```python
from build123d import *

# Parameters (mm, degrees)
SKETCH1_W                = 114.3
SKETCH1_H                = 101.6
BOSS_EXTRUDE1_DEPTH      = 3.175
F_5_16_CLEARANCE_HOLE2_D = 8.4328


with BuildPart() as part:
    # Sketch1 → Boss-Extrude1 (new body)
    with BuildSketch(Plane(origin=(0, 0, 0), x_dir=(1, 0, 0), z_dir=(0, 1, 0))):
        Rectangle(SKETCH1_W, SKETCH1_H)
    extrude(amount=BOSS_EXTRUDE1_DEPTH)

    # 5/16 Clearance Hole2 (through all)
    with Locations(Plane(origin=(0, 3.175, 0), x_dir=(1, 0, 0), z_dir=(0, 1, 0))):
        with Locations((-38.1, 31.75), (-38.1, 0), (-38.1, -34.925)):
            f_5_16_clearance_hole2 = Hole(F_5_16_CLEARANCE_HOLE2_D / 2)

    # Mirror2: 5/16 Clearance Hole2 across plane
    add(f_5_16_clearance_hole2.mirror(Plane(origin=(0, 0, 0), x_dir=(0, 0, 1), z_dir=(1, 0, 0))), mode=Mode.SUBTRACT)


solid = part.part
```
Build history of the part. All positions in model axes, mm. Round coordinates to 2 decimals unless told otherwise and drop trailing zeros. Order: outer loops, then holes, each group sorted by start corner. A loop starts at its lowest first (then second) coordinate and runs counter-clockwise, first axis right, second up. Notation, with made-up numbers: (-35, -26.75) -> (-13, -26.75) arc R19 ccw to (-13, -8.75) -> close; hole circle Ø3 at (53.25, 86.5). An arc over 180 degrees is marked (long way). Answer in a Markdown table with one row per item.
1) Wall check: L1, parallel to Z at x = -38.1, y = 2.1; L2, parallel to X at y = 2.1, z = -28.5; L3, parallel to X at y = 2.6, z = 38. Give the ranges that are in metal, low to high.
Values:
| item | result |
|---|---|
| L1 | -50.8 to -35.97, -27.53 to -4.22, 4.22 to 30.71, 39.14 to 50.8 |
| L2 | -57.15 to -40.79, -35.41 to 35.41, 40.79 to 57.15 |
| L3 | -57.15 to -40.98, -35.22 to 35.22, 40.98 to 57.15 |
2) Band-saw the part on A-A on z = 0. Give the cut face in (x, y) (3 decimals), and give its area (3 significant figures).
Values:
| item | result |
|---|---|
| outline | (-57.15, 0) -> (-42.316, 0) -> (-42.316, 3.175) -> (-57.15, 3.175) -> close; (-33.884, 0) -> (33.884, 0) -> (33.884, 3.175) -> (-33.884, 3.175) -> close; (42.316, 0) -> (57.15, 0) -> (57.15, 3.175) -> (42.316, 3.175) -> close |
| area | 309 mm2 |
3) Band-saw the part on C-C on y = 2.6. Give the cut face in (x, z) (3 decimals).
Values:
| item | result |
|---|---|
| outline | (-57.15, -50.8) -> (57.15, -50.8) -> (57.15, 50.8) -> (-57.15, 50.8) -> close; hole circle Ø8.433 at (-38.1, -31.75); hole circle Ø8.433 at (-38.1, 0); hole circle Ø8.433 at (-38.1, 34.925); hole circle Ø8.433 at (38.1, -31.75); hole circle Ø8.433 at (38.1, 0); hole circle Ø8.433 at (38.1, 34.925) |
4) Mould opens along X. For faces 1 (the cylindrical face through (-42.12, 1.57, -1.27)), 2 (the flat face through (-1, 3.175, -1)), 3 (the cylindrical face through (42.12, 1.57, -1.27)), 4 (the flat face through (57.15, 2, 1)) say: released by +X, released by -X, zero draft, split by the parting line, or undercut.
Values:
| item | result |
|---|---|
| face 1 | undercut |
| face 2 | zero draft |
| face 3 | undercut |
| face 4 | released by +X |
5) Band-saw the part on D-D on z = 36.5. Give the cut face in (x, y) (3 decimals).
Values:
| item | result |
|---|---|
| outline | (-57.15, 0) -> (-42.011, 0) -> (-42.011, 3.175) -> (-57.15, 3.175) -> close; (-34.189, 0) -> (34.189, 0) -> (34.189, 3.175) -> (-34.189, 3.175) -> close; (42.011, 0) -> (57.15, 0) -> (57.15, 3.175) -> (42.011, 3.175) -> close |
6) Pin check, flat tips, straight feed: P1, Ø6.5, axis at x = 38.1, z = -31.75, coming from the -Y side; P2, Ø13.5, axis at x = -38.1, z = 0, coming from the +Y side (3 decimals). Stop position of each tip, or through.
Values:
| item | result |
|---|---|
| P1 | through |
| P2 | y = 3.175 |
7) Band-saw the part on B-B on x = 38.1. Give the cut face in (y, z) (3 decimals).
Values:
| item | result |
|---|---|
| outline | (0, -50.8) -> (3.175, -50.8) -> (3.175, -35.966) -> (0, -35.966) -> close; (0, -27.534) -> (3.175, -27.534) -> (3.175, -4.216) -> (0, -4.216) -> close; (0, 4.216) -> (3.175, 4.216) -> (3.175, 30.709) -> (0, 30.709) -> close; (0, 39.141) -> (3.175, 39.141) -> (3.175, 50.8) -> (0, 50.8) -> close |
